from build123d import *

# Parameters (mm, degrees)
BOSS_EXTRUDE1_DEPTH = 1.5875
SKETCH2_R           = 4.12
SKETCH2_W           = 10
SKETCH2_H           = 3.01
CUT_EXTRUDE1_DEPTH  = 1.5875


with BuildPart() as part:
    # Sketch1 → Boss-Extrude1 (new body)
    with BuildSketch(Plane(origin=(0, 0, 0), x_dir=(0, 0, -1), z_dir=(1, 0, 0))):
        Polygon((0, 17.849301165), (0, 30), (125, 30), (125, -20), (0, 0), (0, 4.461317534), (0, 9.461317534), align=None)
    extrude(amount=BOSS_EXTRUDE1_DEPTH)

    # Sketch2 → Cut-Extrude1 (cut)
    with BuildSketch(Plane(origin=(1.5875, 0, 0), x_dir=(0, 0, -1), z_dir=(1, 0, 0))):
        with Locations((114.49, 10.38)):
            Circle(SKETCH2_R)
        with Locations((54.49, 5.005)):
            Rectangle(SKETCH2_W, SKETCH2_H)
    extrude(amount=-CUT_EXTRUDE1_DEPTH, mode=Mode.SUBTRACT)


solid = part.part
Design review of the part built by this model. Coordinates are the model's own, in mm. Give positions to 0.01 mm unless a question says otherwise; leave off trailing zeros. Loops run counter-clockwise (first coordinate to the right, second up) from the corner with the lowest first, then second, coordinate; pieces in that order, holes last. Notation, with made-up numbers: (71, -19) - (98, -19) arc R9 ccw to (98, -15) - close; hole circle Ø4 at (57.25, 27). An arc over 180 degrees is marked (long way). Use CSV: the item, a comma, the result in double quotes. Start each with the question number.
1. Draft analysis for pull direction Z (two halves, no side actions). For faces 1 (the flat face through (0.78, -10.14, -63.37)), 2 (the flat face through (1.588, 11, -63)), 3 (the cylindrical face through (0.805, 10.561, -110.374)), state which applies: released by +Z, released by -Z, zero draft, split by the parting line, or undercut.
2. Add section A-A (z = -54). State the section outline as (x, y) points.
3. Add section D-D (y = -13). State the section outline as (x, z) points.
4. Add section B-B (x = 0.5). State the section outline as (y, z) points.
5. Insertion check: P1, Ø9.5, axis at y = 10.38, z = -114.49, coming from the +X side; P2, Ø0.5, axis at x = 0.5, z = -55, coming from the -Y side. Each pin has a flat end and moves straight along its axis. Give the tip position at first contact, or say it passes through.
6. Add section C-C (y = 10.38). State the section outline as (x, z) points.
7. Wall thickness on L1, parallel to Y at x = 1.3, z = -114.49; L2, parallel to Y at x = 0.1, z = -51.5; L3, parallel to Y at x = 0.35, z = -60.5: over which ranges is each line inside the solid? List them lowest first.
Results found:
1,face 1,"released by +Z"
1,face 2,"zero draft"
1,face 3,"undercut"
2,outline,"(0, -8.64) - (1.59, -8.64) - (1.59, 3.5) - (0, 3.5) - close; (0, 6.51) - (1.59, 6.51) - (1.59, 30) - (0, 30) - close"
3,outline,"(0, -125) - (1.59, -125) - (1.59, -81.25) - (0, -81.25) - close"
4,outline,"(-20, -125) - (30, -125) - (30, 0) - (0, 0) - close; hole (3.5, -59.49) - (6.51, -59.49) - (6.51, -49.49) - (3.5, -49.49) - close; hole circle Ø8.24 at (10.38, -114.49)"
5,P1,"stops at x = 1.59"
5,P2,"stops at y = -8.84"
6,outline,"(0, -125) - (1.59, -125) - (1.59, -118.61) - (0, -118.61) - close; (0, -110.37) - (1.59, -110.37) - (1.59, 0) - (0, 0) - close"
7,L1,"y = -18.32 to 6.26, 14.5 to 30"
7,L2,"y = -8.24 to 3.5, 6.51 to 30"
7,L3,"y = -9.68 to 30"
